The listing builds one solid part. Answer for the finished solid, in the listing's coordinates (mm). Coordinates: 2 decimals unless noted, no trailing zeros. Order: outer loops, then holes, each group sorted by start corner. A loop starts at its lowest first (then second) coordinate and runs counter-clockwise, first axis right, second up. Notation, with made-up numbers: (37, 67.25) - (96, 67.25) arc R26 ccw to (96, 87.25) - close; hole circle Ø1 at (-5.5, -38.5). An arc over 180 degrees is marked (long way). Use a Markdown table: item, result. Add a question column.
Item 1: The part is cut by section C-C, the plane x = -343. Give the vertices of the cut face in (y, z).
Item 2: Find the intervals of material crossed by line 1 along X through (y, z) = (-123.5, 3.5); line 2 along Y through (x, z) = (-82, 6); line 3 along X through (y, z) = (-78, 1.5), in increasing order.
Item 3: The part is cut by section A-A, the plane y = -61. Give the vertices of the cut face in (x, z), then the cut area to 3 significant figures.
Item 4: Flat-ended cylindrical pins translate along their axes: P1, Ø1, axis at x = -360, z = 6, coming from the +Y side; P2, Ø5, axis at y = -70, z = 2.5, coming from the +X side; P3, Ø6, axis at y = -76.5, z = 7.5, coming from the -X side. Find the tip coordinate at first contact, or state that the pin passes through.
Item 5: The part is cut by section B-B, the plane z = 5.5. Give the vertices of the cut face in (x, y).
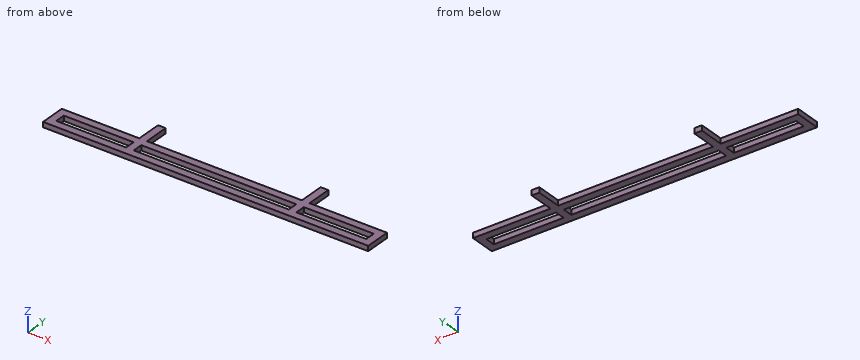
from build123d import *

# Parameters (mm, degrees)
SKETCH1_W                = 640
SKETCH1_H                = 50
BOSS_EXTRUDE1_DEPTH      = 10
SKETCH2_W                = 15
SKETCH2_H                = 50
BOSS_EXTRUDE2_DEPTH      = 10
SKETCH3_W                = 610
SKETCH3_H                = 20
CUT_EXTRUDE1_DEPTH       = 10
ESBO_O1_W                = 15
ESBO_O1_H                = 20
RESSALTO_EXTRUS_O1_DEPTH = 10


with BuildPart() as part:
    # Sketch1 → Boss-Extrude1 (new body)
    with BuildSketch(Plane.XY):
        with Locations((-320, -120.36)):
            Rectangle(SKETCH1_W, SKETCH1_H)
    extrude(amount=BOSS_EXTRUDE1_DEPTH)

    # Sketch2 → Boss-Extrude2 (add)
    with BuildSketch(Plane.XY):
        with Locations((-160, -70.36)):
            Rectangle(SKETCH2_W, SKETCH2_H)
        with Locations((-480, -70.36)):
            Rectangle(SKETCH2_W, SKETCH2_H)
    extrude(amount=BOSS_EXTRUDE2_DEPTH)

    # Sketch3 → Cut-Extrude1 (cut)
    with BuildSketch(Plane(origin=(0, 0, 0), x_dir=(-1, 0, 0), z_dir=(0, 0, -1))):
        with Locations((320, -120.36)):
            Rectangle(SKETCH3_W, SKETCH3_H)
    extrude(amount=-CUT_EXTRUDE1_DEPTH, mode=Mode.SUBTRACT)

    # Esboço1 → Ressalto-extrusão1 (add)
    with BuildSketch(Plane.XY.offset(10)):
        with Locations((-480, -120.36)):
            Rectangle(ESBO_O1_W, ESBO_O1_H)
        with Locations((-160, -120.36)):
            Rectangle(ESBO_O1_W, ESBO_O1_H)
    extrude(amount=-RESSALTO_EXTRUS_O1_DEPTH)


solid = part.part
Solution:
| question | item | result |
|---|---|---|
| 1 | outline | (-145.36, 0) - (-130.36, 0) - (-130.36, 10) - (-145.36, 10) - close; (-110.36, 0) - (-95.36, 0) - (-95.36, 10) - (-110.36, 10) - close |
| 2 | line 1 | x = -640 to -625, -487.5 to -472.5, -167.5 to -152.5, -15 to 0 |
| 2 | line 2 | y = -145.36 to -130.36, -110.36 to -95.36 |
| 2 | line 3 | x = -487.5 to -472.5, -167.5 to -152.5 |
| 3 | outline | (-487.5, 0) - (-472.5, 0) - (-472.5, 10) - (-487.5, 10) - close; (-167.5, 0) - (-152.5, 0) - (-152.5, 10) - (-167.5, 10) - close |
| 3 | area | 300 mm2 |
| 4 | P1 | stops at y = -95.36 |
| 4 | P2 | stops at x = -152.5 |
| 4 | P3 | stops at x = -487.5 |
| 5 | outline | (-640, -145.36) - (0, -145.36) - (0, -95.36) - (-152.5, -95.36) - (-152.5, -45.36) - (-167.5, -45.36) - (-167.5, -95.36) - (-472.5, -95.36) - (-472.5, -45.36) - (-487.5, -45.36) - (-487.5, -95.36) - (-640, -95.36) - close; hole (-625, -130.36) - (-487.5, -130.36) - (-487.5, -110.36) - (-625, -110.36) - close; hole (-472.5, -130.36) - (-167.5, -130.36) - (-167.5, -110.36) - (-472.5, -110.36) - close; hole (-152.5, -130.36) - (-15, -130.36) - (-15, -110.36) - (-152.5, -110.36) - close |
